```python
from build123d import *

# Parameters (mm, degrees)
SKETCH1_W           = 26.02
SKETCH1_H           = 19.02
SKETCH1_W_2         = 23.02
SKETCH1_H_2         = 16.02
BOSS_EXTRUDE1_DEPTH = 11.5
SKETCH2_W           = 26.02
SKETCH2_H           = 19.02
SKETCH2_W_2         = 21.02
SKETCH2_H_2         = 14.02
BOSS_EXTRUDE2_DEPTH = 1.5
SKETCH3_W           = 26.02
SKETCH3_H           = 19.02
SKETCH3_R           = 4.1
BOSS_EXTRUDE3_DEPTH = 1.5
SKETCH4_R           = 5.6
SKETCH4_R_2         = 4.1
BOSS_EXTRUDE4_DEPTH = 2
BOSS_EXTRUDE4_DRAFT = 5
SKETCH5_R           = 3
CUT_EXTRUDE1_DEPTH  = 1.5
CUT_EXTRUDE2_DEPTH  = 29.343261986


with BuildPart() as part:
    # Sketch1 → Boss-Extrude1 (new body)
    with BuildSketch(Plane.XY):
        with Locations((3.5, 0)):
            Rectangle(SKETCH1_W, SKETCH1_H)
        with Locations((3.5, 0)):
            Rectangle(SKETCH1_W_2, SKETCH1_H_2, mode=Mode.SUBTRACT)
    extrude(amount=-BOSS_EXTRUDE1_DEPTH)

    # Sketch2 → Boss-Extrude2 (add)
    with BuildSketch(Plane(origin=(0, 0, -11.5), x_dir=(-1, 0, 0), z_dir=(0, 0, -1))):
        with Locations((-3.5, 0)):
            Rectangle(SKETCH2_W, SKETCH2_H)
        with Locations((-3.5, 0)):
            Rectangle(SKETCH2_W_2, SKETCH2_H_2, mode=Mode.SUBTRACT)
    extrude(amount=BOSS_EXTRUDE2_DEPTH)

    # Sketch3 → Boss-Extrude3 (add)
    with BuildSketch(Plane.XY):
        with Locations((3.5, 0)):
            Rectangle(SKETCH3_W, SKETCH3_H)
        Circle(SKETCH3_R, mode=Mode.SUBTRACT)
    extrude(amount=BOSS_EXTRUDE3_DEPTH)


with BuildPart() as boss_extrude4_tool:
    # Sketch4 → Boss-Extrude4 (with draft: the straight prism first)
    with BuildSketch(Plane.XY.offset(1.5)):
        Circle(SKETCH4_R)
        Circle(SKETCH4_R_2, mode=Mode.SUBTRACT)
    extrude(amount=BOSS_EXTRUDE4_DEPTH)
    # Boss-Extrude4: the draft: its side faces are tilted about the plane it starts from
    boss_extrude4_sides = [boss_extrude4_tool.faces().sort_by_distance(p)[0] for p in [
        (-5.6, 0, 2.5),
        (-4.1, 0, 2.5),
    ]]
    draft(boss_extrude4_sides, Plane.XY.offset(1.5), BOSS_EXTRUDE4_DRAFT)


with BuildPart() as part_1:
    add(part.part)

    # Boss-Extrude4: add boss_extrude4_tool
    add(boss_extrude4_tool.part)

    # Sketch5 → Cut-Extrude1 (cut)
    with BuildSketch(Plane.XY.offset(1.5)):
        with Locations((12.502526503, 1e-09)):
            Circle(SKETCH5_R)
    extrude(amount=-CUT_EXTRUDE1_DEPTH, mode=Mode.SUBTRACT)

    # Sketch6 → Cut-Extrude2 (cut, through all)
    with BuildSketch(Plane.XZ.offset(9.51)):
        with BuildLine():
            Line((3.375, -4), (3.375, -13))
            Line((3.375, -13), (9.625, -13))
            Line((9.625, -13), (9.625, -4))
            ThreePointArc((9.625, -4), (6.5, -0.875), (3.375, -4))
        make_face()
        with BuildLine():
            Line((-4.25, -5.75), (-4.25, -13))
            Line((-4.25, -13), (-7.75, -13))
            Line((-7.75, -13), (-7.75, -5.75))
            ThreePointArc((-7.75, -5.75), (-6, -4), (-4.25, -5.75))
        make_face()
    extrude(amount=-CUT_EXTRUDE2_DEPTH, mode=Mode.SUBTRACT)


solid = part_1.part
```
Build history of the part. All positions in model axes, mm. A direction names the side the tool comes from. Coordinates: 2 decimals unless noted, no trailing zeros. Order: outer loops, then holes, each group sorted by start corner. A loop starts at its lowest first (then second) coordinate and runs counter-clockwise, first axis right, second up. Notation, with made-up numbers: (-3.5, 33.25) -> (14.5, 33.25) arc R18 ccw to (14.5, 40.25) -> close; hole circle Ø8 at (50, -19.75). An arc over 180 degrees is marked (long way). Answer in a Markdown table with one row per item. Add a question column.
Q1. Mould opens along Y. For faces 1 (the face through (-4.25, -9, -10)), 2 (the face through (0, 7.01, -12)), 3 (the face through (-8.01, 0, -6)), 4 (the face through (3, -9.51, -6)) say: +Y half, -Y half, draft (parallel to the pull), parting line (faces both ways), or undercut.
Q2. Band-saw the part on D-D, the plane y = 6.25. List the corners of the cut face in (x, z).
Q3. Band-saw the part on C-C, the plane x = -6. List the corners of the cut face in (y, z), then the cut area to 3 significant figures.
Q4. Band-saw the part on A-A, the plane z = -9. List the corners of the cut face in (x, y) (3 decimals), then the cut area to 3 significant figures.
Q5. Which spindle directions (+Z, -Z, +X, -X, +Y, -Y) get a long thin tool onto all of the face, cutting with end or side? Do faces 5 (the face through (3, 9.51, -6)), 6 (the face through (-0.4, -7.5, -11.5)), 7 (the face through (6, 0, 1.5)), 8 (the face through (12, 7.01, -12)), 9 (the face through (3.375, -9, -8)). Say none if no direction does.
Q6. Band-saw the part on B-B, the plane y = 0. List the corners of the cut face in (x, z), then the cut area to 3 significant figures.
Q7. Wall check: line 1 along X through (y, z) = (4, -10); line 2 along Y through (x, z) = (12.5, -8); line 3 along Y through (x, z) = (0, 0.3). Give the ranges that are in metal, low to high. Write a range as [from, to].
Q8. Drop flat-ended pins along their axis: pin 1 (5.5 mm diameter, centred on x = 12.5, y = 0, fed in from +Z); pin 2 (6 mm diameter, centred on x = 12, y = 2, fed in from +Z); pin 3 (1 mm diameter, centred on x = 11, y = -5, fed in from -Z). Give the stop position or say it passes through.
Answers follow:
| question | item | result |
|---|---|---|
| 1 | face 1 | draft |
| 1 | face 2 | undercut |
| 1 | face 3 | undercut |
| 1 | face 4 | -Y half |
| 2 | outline | (-9.51, -13) -> (-7.75, -13) -> (-7.75, -11.5) -> (-8.01, -11.5) -> (-8.01, 0) -> (15.01, 0) -> (15.01, -11.5) -> (14.01, -11.5) -> (14.01, -13) -> (16.51, -13) -> (16.51, 1.5) -> (-9.51, 1.5) -> close |
| 3 | outline | (-9.51, -4) -> (-8.01, -4) -> (-8.01, 0) -> (8.01, 0) -> (8.01, -4) -> (9.51, -4) -> (9.51, 1.5) -> (-9.51, 1.5) -> close |
| 3 | area | 40.5 mm^2 |
| 4 | outline | (-9.51, -9.51) -> (-7.75, -9.51) -> (-7.75, -8.01) -> (-8.01, -8.01) -> (-8.01, 8.01) -> (-7.75, 8.01) -> (-7.75, 9.51) -> (-9.51, 9.51) -> close; (-4.25, -9.51) -> (3.375, -9.51) -> (3.375, -8.01) -> (-4.25, -8.01) -> close; (-4.25, 8.01) -> (3.375, 8.01) -> (3.375, 9.51) -> (-4.25, 9.51) -> close; (9.625, -9.51) -> (16.51, -9.51) -> (16.51, 9.51) -> (9.625, 9.51) -> (9.625, 8.01) -> (15.01, 8.01) -> (15.01, -8.01) -> (9.625, -8.01) -> close |
| 4 | area | 96.9 mm^2 |
| 5 | face 5 | +Z, -Z, +X, -X, +Y |
| 5 | face 6 | none |
| 5 | face 7 | +Z |
| 5 | face 8 | -Z |
| 5 | face 9 | -Z, +Y, -Y |
| 6 | outline | (-9.51, -13) -> (-7.75, -13) -> (-7.75, -11.5) -> (-8.01, -11.5) -> (-8.01, 0) -> (-4.1, 0) -> (-4.1, 1.5) -> (-4.27, 3.5) -> (-5.43, 3.5) -> (-5.6, 1.5) -> (-9.51, 1.5) -> close; (4.1, 0) -> (9.5, 0) -> (9.5, 1.5) -> (5.6, 1.5) -> (5.43, 3.5) -> (4.27, 3.5) -> (4.1, 1.5) -> close; (14.01, -13) -> (16.51, -13) -> (16.51, 1.5) -> (15.5, 1.5) -> (15.5, 0) -> (15.01, 0) -> (15.01, -11.5) -> (14.01, -11.5) -> close |
| 6 | area | 63.9 mm^2 |
| 7 | line 1 | [-9.51, -8.01], [15.01, 16.51] |
| 7 | line 2 | [-9.51, -8.01], [8.01, 9.51] |
| 7 | line 3 | [-9.51, -4.1], [4.1, 9.51] |
| 8 | pin 1 | z = 0 |
| 8 | pin 2 | z = 1.5 |
| 8 | pin 3 | z = 0 |
